```python
from build123d import *

# Parameters (mm, degrees)
SKETCH2_R           = 3
SKETCH2_R_2         = 2
BOSS_EXTRUDE1_DEPTH = 3
SKETCH2_3_R         = 3
SKETCH2_3_R_2       = 2
BOSS_EXTRUDE2_DEPTH = 12
SKETCH3_R           = 2
BOSS_EXTRUDE3_DEPTH = 4


with BuildPart() as part:
    # Sketch2 → Boss-Extrude1 (new body)
    # profile 1 of 3: a face of its own
    with BuildSketch(Plane(origin=(0, 0, 0), x_dir=(0, 0, -1), z_dir=(1, 0, 0))):
        with BuildLine():
            Line((3.31662479, -5), (-3.31662479, -5))
            ThreePointArc((-3.31662479, -5), (-6, 0), (-3.31662479, 5))
            Line((-3.31662479, 5), (3.31662479, 5))
            ThreePointArc((3.31662479, 5), (6, 0), (3.31662479, -5))
        make_face()
        Circle(SKETCH2_R, mode=Mode.SUBTRACT)
    # profile 2 of 3: a face of its own
    with BuildSketch(Plane(origin=(0, 0, 0), x_dir=(0, 0, -1), z_dir=(1, 0, 0))):
        Circle(SKETCH2_R)
        Circle(SKETCH2_R_2, mode=Mode.SUBTRACT)
    # profile 3 of 3: a face of its own
    with BuildSketch(Plane(origin=(0, 0, 0), x_dir=(0, 0, -1), z_dir=(1, 0, 0))):
        Circle(SKETCH2_R_2)
    extrude(amount=BOSS_EXTRUDE1_DEPTH)

    # Sketch2_3 → Boss-Extrude2 (add)
    # profile 1 of 2: a face of its own
    with BuildSketch(Plane(origin=(0, 0, 0), x_dir=(0, 0, -1), z_dir=(1, 0, 0))):
        Circle(SKETCH2_3_R)
        Circle(SKETCH2_3_R_2, mode=Mode.SUBTRACT)
    # profile 2 of 2: a face of its own
    with BuildSketch(Plane(origin=(0, 0, 0), x_dir=(0, 0, -1), z_dir=(1, 0, 0))):
        Circle(SKETCH2_3_R_2)
    extrude(amount=-BOSS_EXTRUDE2_DEPTH)

    # Sketch3 → Boss-Extrude3 (add)
    with BuildSketch(Plane.ZY.offset(12)):
        Circle(SKETCH3_R)
    extrude(amount=BOSS_EXTRUDE3_DEPTH)


solid = part.part
```
CAD build for the part. Positions are in the model's coordinates, mm. A direction names the side the tool comes from. Give positions to 0.01 mm unless a question says otherwise; leave off trailing zeros. Write each loop counter-clockwise with the first axis right and the second up, starting at its lowest first coordinate (ties: lowest second). Pieces come first, ordered by that corner, then holes. Notation, with made-up numbers: M -37,-35 L 13,-35 A12 cw 13,-20 Z; hole C -29,7.5 d8. An arc over 180 degrees is marked long. Return JSON: item names as keys, results as strings. Group by question number.
(1) Drill centre lines: L1, parallel to X at y = -2, z = 4.5; L2, parallel to X at y = 1.75, z = 2; L3, parallel to Z at x = -7, y = 2.75. Where is each one in solid material? Low to high. Write a range as [from, to].
(2) 3-axis set-ups, long thin cutter, end or side, ignore diameter. For faces 4 (the face through (3, 0, 0)), 5 (the face through (-14, -2, 0)): which of +Z, -Z, +X, -X, +Y, -Y reach the whole face in a straight line?
(3) Band-saw the part on D-D (z = 5.25). Give the cut face in (x, y).
(4) Flat gauge pins, fed straight in: pin 1 Ø1.5 at (x, y) = (-10, 3) entering from -Z; pin 2 Ø1.5 at (x, z) = (-4, -1) entering from -Y; pin 3 Ø5 at (x, z) = (-3.5, -4) entering from -Y. Where does each tip first touch, or does it go through?
(5) Band-saw the part on C-C (x = -4.5). Give the cut face in (y, z).
(6) Mould opens along Y. For faces 1 (the face through (1, 0, -6)), 2 (the face through (-12, -2, -1)), 3 (the face through (1, 5, 0)) say: pulls with the +Y half, pulls with the -Y half, needs draft (parallel to the pull), parting line crosses it, or undercut.
(7) Band-saw the part on B-B (y = 0). Give the cut face in (x, z), and give its area (3 significant figures).
(8) Band-saw the part on A-A (z = 0). Give the cut face in (x, y).
Entries:
{
 "1": {"L1": "x = [0, 3]", "L2": "x = [-12, 3]", "L3": "z = [-1.2, 1.2]"},
 "2": {"face 4": "+Z, -Z, +X, +Y, -Y", "face 5": "-X"},
 "3": {"outline": "M 0,-2.9 L 3,-2.9 L 3,2.9 L 0,2.9 Z"},
 "4": {"pin 1": "stops at z = -1.98", "pin 2": "stops at y = -2.99", "pin 3": "stops at y = -2.6"},
 "5": {"outline": "C 0,0 d6"},
 "6": {"face 1": "parting line crosses it", "face 2": "needs draft", "face 3": "pulls with the +Y half"},
 "7": {"outline": "M -16,-2 L -12,-2 L -12,-3 L 0,-3 L 0,-6 L 3,-6 L 3,6 L 0,6 L 0,3 L -12,3 L -12,2 L -16,2 Z", "area": "124 mm^2"},
 "8": {"outline": "M -16,-2 L -12,-2 L -12,-3 L 0,-3 L 0,-5 L 3,-5 L 3,5 L 0,5 L 0,3 L -12,3 L -12,2 L -16,2 Z"}
}
